```python
from build123d import *

# Parameters (mm, degrees)
F0_W      = 27.8634205461
F0_H      = 28.4682586789
F1_DEPTH  = 25.4
F2_W      = 3.9148032665
F2_H      = 3.3797924407
F3_DEPTH  = 50.8
F4_W      = 3.8050059229
F4_H      = 3.4576065373
F5_DEPTH  = 50.8
F6_W      = 3.416453721
F6_H      = 3.6132577807
F7_DEPTH  = 50.8
F9_W      = 3.0085314065
F9_H      = 3.2848082483
F10_DEPTH = 50.8
F8_W      = 4.4579515234
F8_H      = 27.902291331
F11_DEPTH = 50.8
F12_W     = 2.1538413306
F12_H     = 14.2136927884
F13_DEPTH = 2.54


with BuildPart() as f1:
    # F0 (on Front) → F1 (new body)
    with BuildSketch(Plane.XZ):
        with Locations((-13.931710273, -14.2341293395)):
            Rectangle(F0_W, F0_H)
    extrude(amount=F1_DEPTH)

    # F2 (on face) → F3 (join)
    with BuildSketch(Plane(origin=(-27.8634205461, 0, 0), x_dir=(0, -1, 0), z_dir=(-1, 0, 0))):
        with Locations((3.7574605085, -4.493831424)):
            Rectangle(F2_W, F2_H)
    extrude(amount=F3_DEPTH)

    # F4 (on face) → F5 (join)
    with BuildSketch(Plane(origin=(-27.8634205461, 0, 0), x_dir=(0, -1, 0), z_dir=(-1, 0, 0))):
        with Locations((20.2637864277, -3.7950236583)):
            Rectangle(F4_W, F4_H)
    extrude(amount=F5_DEPTH)

    # F6 (on face) → F7 (join)
    with BuildSketch(Plane(origin=(-27.8634205461, 0, 0), x_dir=(0, -1, 0), z_dir=(-1, 0, 0))):
        with Locations((4.1821881896, -24.0737376735)):
            Rectangle(F6_W, F6_H)
    extrude(amount=F7_DEPTH)

    # F9 (on face) → F10 (join)
    with BuildSketch(Plane(origin=(-27.8634205461, 0, 0), x_dir=(0, -1, 0), z_dir=(-1, 0, 0))):
        with Locations((22.4483674392, -22.9268092662)):
            Rectangle(F9_W, F9_H)
    extrude(amount=F10_DEPTH)

    # F8 (on face) → F11 (join)
    with BuildSketch(Plane.YZ):
        with Locations((-2.2289757617, -14.5171130134)):
            Rectangle(F8_W, F8_H)
    extrude(amount=F11_DEPTH)

    # F12 (on face) → F13 (join)
    with BuildSketch(Plane(origin=(0, 0, 0), x_dir=(-1, 0, 0), z_dir=(0, 1, 0))):
        Polygon((27.8634205461, 0), (0, 0), (0, -0.5659673479), (-50.8, -0.5659673479), (-50.8, -28.4682586789), (27.8634205461, -28.4682586789), align=None)
        with BuildLine():
            add(Edge.make_bspline(
                [(-14.5633904309, -24.9638148742), (-15.5801363384, -25.1796140055), (-17.0201805421, -25.1796140055)],
                knots=[0, 0, 0, 1, 1, 1], degree=2))
            add(Edge.make_bspline(
                [(-17.0201805421, -25.1796140055), (-20.1700178637, -25.1796140055), (-21.9939355222, -23.2581717395)],
                knots=[0, 0, 0, 1, 1, 1], degree=2))
            add(Edge.make_bspline(
                [(-21.9939355222, -23.2581717395), (-23.8178531807, -21.3367294736), (-23.8178531807, -17.9295931876)],
                knots=[0, 0, 0, 1, 1, 1], degree=2))
            add(Edge.make_bspline(
                [(-23.8178531807, -17.9295931876), (-23.8178531807, -14.4892570354), (-22.124659996, -12.4661401786)],
                knots=[0, 0, 0, 1, 1, 1], degree=2))
            add(Edge.make_bspline(
                [(-22.124659996, -12.4661401786), (-20.4314668113, -10.4430233219), (-17.5762783037, -10.4430233219)],
                knots=[0, 0, 0, 1, 1, 1], degree=2))
            add(Edge.make_bspline(
                [(-17.5762783037, -10.4430233219), (-14.9078390445, -10.4430233219), (-13.3515953086, -12.2005412477)],
                knots=[0, 0, 0, 1, 1, 1], degree=2))
            add(Edge.make_bspline(
                [(-13.3515953086, -12.2005412477), (-11.7953515726, -13.9580591735), (-11.7953515726, -16.8381475808)],
                knots=[0, 0, 0, 1, 1, 1], degree=2))
            Line((-11.7953515726, -16.8381475808), (-11.7953515726, -18.1993421019))
            Line((-11.7953515726, -18.1993421019), (-21.5851621676, -18.1993421019))
            add(Edge.make_bspline(
                [(-21.5851621676, -18.1993421019), (-21.5187624348, -20.7017820293), (-20.3194172623, -21.9986518093)],
                knots=[0, 0, 0, 1, 1, 1], degree=2))
            add(Edge.make_bspline(
                [(-20.3194172623, -21.9986518093), (-19.1200720898, -23.2955215892), (-16.9413308595, -23.2955215892)],
                knots=[0, 0, 0, 1, 1, 1], degree=2))
            add(Edge.make_bspline(
                [(-16.9413308595, -23.2955215892), (-14.6463900969, -23.2955215892), (-12.4053991171, -22.3368754479)],
                knots=[0, 0, 0, 1, 1, 1], degree=2))
            Line((-12.4053991171, -22.3368754479), (-12.4053991171, -24.2583177139))
            add(Edge.make_bspline(
                [(-12.4053991171, -24.2583177139), (-13.5466445235, -24.7480157428), (-14.5633904309, -24.9638148742)],
                knots=[0, 0, 0, 1, 1, 1], degree=2))
        make_face(mode=Mode.SUBTRACT)
        with BuildLine():
            Line((-25.6189459312, -10.7044722695), (-25.6189459312, -12.3769155378))
            Line((-25.6189459312, -12.3769155378), (-29.2377313652, -12.3769155378))
            Line((-29.2377313652, -12.3769155378), (-29.2377313652, -24.9181650579))
            Line((-29.2377313652, -24.9181650579), (-31.3915726957, -24.9181650579))
            Line((-31.3915726957, -24.9181650579), (-31.3915726957, -12.3769155378))
            Line((-31.3915726957, -12.3769155378), (-33.9313624728, -12.3769155378))
            Line((-33.9313624728, -12.3769155378), (-33.9313624728, -11.4058194465))
            Line((-33.9313624728, -11.4058194465), (-31.3915726957, -10.6256225869))
            Line((-31.3915726957, -10.6256225869), (-31.3915726957, -9.8371257607))
            add(Edge.make_bspline(
                [(-31.3915726957, -9.8371257607), (-31.3915726957, -4.595696858), (-26.8141411204, -4.595696858)],
                knots=[0, 0, 0, 1, 1, 1], degree=2))
            add(Edge.make_bspline(
                [(-26.8141411204, -4.595696858), (-25.6853456639, -4.595696858), (-24.1664517776, -5.0480450373)],
                knots=[0, 0, 0, 1, 1, 1], degree=2))
            Line((-24.1664517776, -5.0480450373), (-24.7266995225, -6.7744380883))
            add(Edge.make_bspline(
                [(-24.7266995225, -6.7744380883), (-25.9716945113, -6.3718897086), (-26.85149097, -6.3718897086)],
                knots=[0, 0, 0, 1, 1, 1], degree=2))
            add(Edge.make_bspline(
                [(-26.85149097, -6.3718897086), (-28.071586059, -6.3718897086), (-28.6546587121, -7.183211443)],
                knots=[0, 0, 0, 1, 1, 1], degree=2))
            add(Edge.make_bspline(
                [(-28.6546587121, -7.183211443), (-29.2377313652, -7.9945331773), (-29.2377313652, -9.7831759778)],
                knots=[0, 0, 0, 1, 1, 1], degree=2))
            Line((-29.2377313652, -9.7831759778), (-29.2377313652, -10.7044722695))
            Line((-29.2377313652, -10.7044722695), (-25.6189459312, -10.7044722695))
        make_face(mode=Mode.SUBTRACT)
        with Locations((-7.0456956905, -17.8113186637)):
            Rectangle(F12_W, F12_H, mode=Mode.SUBTRACT)
        with BuildLine():
            add(Edge.make_bspline(
                [(-7.9420920824, -7.9364334112), (-8.3052156208, -7.5795348477), (-8.3052156208, -6.853287771)],
                knots=[0, 0, 0, 1, 1, 1], degree=2))
            add(Edge.make_bspline(
                [(-8.3052156208, -6.853287771), (-8.3052156208, -6.1145907443), (-7.9420920824, -5.7701421307)],
                knots=[0, 0, 0, 1, 1, 1], degree=2))
            add(Edge.make_bspline(
                [(-7.9420920824, -5.7701421307), (-7.578968544, -5.4256935172), (-7.0311707489, -5.4256935172)],
                knots=[0, 0, 0, 1, 1, 1], degree=2))
            add(Edge.make_bspline(
                [(-7.0311707489, -5.4256935172), (-6.512422837, -5.4256935172), (-6.1368493487, -5.7763671057)],
                knots=[0, 0, 0, 1, 1, 1], degree=2))
            add(Edge.make_bspline(
                [(-6.1368493487, -5.7763671057), (-5.7612758604, -6.1270406942), (-5.7612758604, -6.853287771)],
                knots=[0, 0, 0, 1, 1, 1], degree=2))
            add(Edge.make_bspline(
                [(-5.7612758604, -6.853287771), (-5.7612758604, -7.5795348477), (-6.1368493487, -7.9364334112)],
                knots=[0, 0, 0, 1, 1, 1], degree=2))
            add(Edge.make_bspline(
                [(-6.1368493487, -7.9364334112), (-6.512422837, -8.2933319746), (-7.0311707489, -8.2933319746)],
                knots=[0, 0, 0, 1, 1, 1], degree=2))
            add(Edge.make_bspline(
                [(-7.0311707489, -8.2933319746), (-7.578968544, -8.2933319746), (-7.9420920824, -7.9364334112)],
                knots=[0, 0, 0, 1, 1, 1], degree=2))
        make_face(mode=Mode.SUBTRACT)
    extrude(amount=F13_DEPTH)


solid = f1.part
```
The listing builds one solid part. Answer for the finished solid, in the listing's coordinates (mm). A direction names the side the tool comes from. Give positions to 0.01 mm unless a question says otherwise; leave off trailing zeros. Write each loop counter-clockwise with the first axis right and the second up, starting at its lowest first coordinate (ties: lowest second). Pieces come first, ordered by that corner, then holes. Notation, with made-up numbers: (66.25, 18.5) - (100.25, 18.5) arc R9 ccw to (100.25, 25.5) - close; hole circle Ø6 at (64, 28). An arc over 180 degrees is marked (long way). Use one line per item in the form item = value. Start each with the question number.
1) Flat-ended cylindrical pins translate along their axes: pin 1 Ø1.3 at (y, z) = (1.5, -20.5) entering from -X; pin 2 Ø1.3 at (x, y) = (16.5, 1) entering from +Z; pin 3 Ø8.5 at (y, z) = (-13.5, -17) entering from +X. Find the tip coordinate at first contact, or state that the pin passes through.
2) A tool of negligible diameter and unlimited length cuts with its end or side. For faces 5 (the face through (-53, -2.474, -24)), 6 (the face through (-53, -20.944, -23)), 7 (the face through (32.68, 1.25, -11.02)), from which of +Z, -Z, +X, -X, +Y, -Y can it reach the whole face along a straight path? Write none if from no direction.
3) Find section B-B on x = 40. Determine the outline of the cut face in (y, z), plus the area to 3 significant figures.
4) Consider line 1 along Y through (x, z) = (-66, -5.25); line 2 along X through (y, z) = (-12, -18.25); line 3 along Z through (x, y) = (-68.5, -5). Determine where each line is inside the solid, lowest interval first. Write a range as from..to.
5) Find section A-A on x = -34.5. Determine the outline of the cut face in (y, z), plus the area to 3 significant figures.
6) Find section C-C on y = -14.25. Determine the outline of the cut face in (x, z).
7) The mould has two halves that part along Z. Classify faces 1 (the face through (25, -1, -0.566)), 2 (the face through (17, 1, -18.199)), 3 (the face through (27, 1, -10.704)), 4 (the face through (-78.663, -4, -24)): pulls with the +Z half, pulls with the -Z half, needs draft (parallel to the pull), parting line crosses it, or undercut.
Geometry results:
q1.pin_1 = -27.86
q1.pin_2 = -0.57
q1.pin_3 = 0
q2.face_5 = -Z, -X, +Y
q2.face_6 = -Z, -X
q2.face_7 = +Y
q3.outline = (-4.46, -28.47) - (2.54, -28.47) - (2.54, -0.57) - (-4.46, -0.57) - close
q3.area = 195 mm2
q4.line_1 = -22.17..-18.36, -5.71..-1.8
q4.line_2 = -27.86..0
q4.line_3 = -25.88..-22.27, -6.18..-2.8
q5.outline = (-23.95, -24.57) - (-20.94, -24.57) - (-20.94, -21.28) - (-23.95, -21.28) - close; (-22.17, -5.52) - (-18.36, -5.52) - (-18.36, -2.07) - (-22.17, -2.07) - close; (-5.89, -25.88) - (-2.47, -25.88) - (-2.47, -22.27) - (-5.89, -22.27) - close; (-5.71, -6.18) - (-1.8, -6.18) - (-1.8, -2.8) - (-5.71, -2.8) - close
q5.area = 48.6 mm2
q6.outline = (-27.86, -28.47) - (0, -28.47) - (0, 0) - (-27.86, 0) - close
q7.face_1 = pulls with the +Z half
q7.face_2 = undercut
q7.face_3 = undercut
q7.face_4 = needs draft
